For this review, take the finished solid that the model builds, in its own axes (mm). Face numbers are marked on the shaded views. A direction names the side the tool comes from. Round coordinates to 2 decimals unless told otherwise and drop trailing zeros. Loops run counter-clockwise (first coordinate to the right, second up) from the corner with the lowest first, then second, coordinate; pieces in that order, holes last.
1) Take a section at D-D (x = 24.5). State the section outline as (y, z) points, then the cut area to 3 significant figures.
2) Take a section at C-C (y = 42.5). State the section outline as (x, z) points.
3) Tool access review of the marked faces 1 and 2: name each direction out of +Z, -Z, +X, -X, +Y, -Y from which nothing blocks a thin tool from reaching the whole face with its end or side.
4) Take a section at A-A (z = 3). State the section outline as (x, y) points, then the cut area to 3 significant figures.
5) Insertion check: pin 1 (1.5 mm diameter, centred on x = 79, y = 78, fed in from +Z); pin 2 (12 mm diameter, centred on x = 22.5, y = 77.5, fed in from +Z). Each pin has a flat end and moves straight along its axis. Give the tip position at first contact, or say it passes through.
6) Take a section at B-B (x = 38). State the section outline as (y, z) points, then the cut area to 3 significant figures.
7) Mouldability with a two-part tool opening along X and no side actions: class the marked faces 3, 4 and 5 as pulls with the +X half, pulls with the -X half, needs draft (parallel to the pull), parting line crosses it, or undercut.
8) Wall thickness on L1, parallel to Y at x = 52, z = 10.25; L2, parallel to X at y = 70, z = 4; L3, parallel to Z at x = 44, y = 64.5: over which ranges is each line inside the solid? List them lowest first.
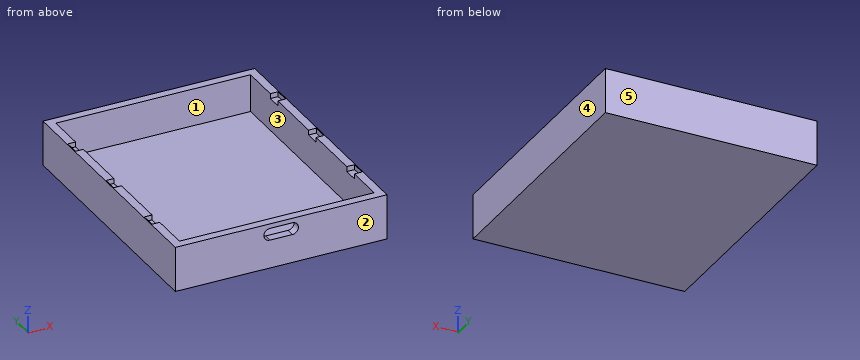
```python
from build123d import *

# Parameters (mm, degrees)
MODEL_W             = 84.74935
MODEL_H             = 103.79946
MODEL_W_2           = 77.94935
MODEL_H_2           = 96.99946
EXTRUDE_2_DEPTH     = 15
SKETCH_1_W          = 84.74935
SKETCH_1_H          = 103.79946
EXTRUDE_3_DEPTH     = 3
SKETCH_2_W          = 3.1
SKETCH_2_H          = 6
CUT_EXTRUDE_1_DEPTH = 2
CUT_EXTRUDE_3_DEPTH = 10


with BuildPart() as part:
    # Model → 凸台-拉伸2 (new body)
    with BuildSketch(Plane.XY):
        with Locations((38.194325, 47.88337)):
            Rectangle(MODEL_W, MODEL_H)
        with Locations((38.194325, 47.88337)):
            Rectangle(MODEL_W_2, MODEL_H_2, mode=Mode.SUBTRACT)
    extrude(amount=EXTRUDE_2_DEPTH)

    # 草图1 → 凸台-拉伸3 (add)
    with BuildSketch(Plane(origin=(0, 0, 0), x_dir=(-1, 0, 0), z_dir=(0, 0, -1))):
        with Locations((-38.194325, 47.88337)):
            Rectangle(SKETCH_1_W, SKETCH_1_H)
    extrude(amount=EXTRUDE_3_DEPTH)

    # 草图2 → 切除-拉伸1 (cut)
    with BuildSketch(Plane.XY.offset(15)):
        with Locations((-2.33035, 77.88337)):
            Rectangle(SKETCH_2_W, SKETCH_2_H)
        with Locations((-2.33035, 47.88337)):
            Rectangle(SKETCH_2_W, SKETCH_2_H)
        with Locations((-2.33035, 17.88337)):
            Rectangle(SKETCH_2_W, SKETCH_2_H)
        with Locations((78.719, 17.88337)):
            Rectangle(SKETCH_2_W, SKETCH_2_H)
        with Locations((78.719, 47.88337)):
            Rectangle(SKETCH_2_W, SKETCH_2_H)
        with Locations((78.719, 77.88337)):
            Rectangle(SKETCH_2_W, SKETCH_2_H)
    extrude(amount=-CUT_EXTRUDE_1_DEPTH, mode=Mode.SUBTRACT)

    # 草图4 → 切除-拉伸3 (cut)
    with BuildSketch(Plane.XZ.offset(7.21636)):
        with BuildLine():
            Line((33.694325, 13.169990539), (42.694325, 13.169990539))
            ThreePointArc((42.694325, 13.169990539), (45.094325, 10.769990539), (42.694325, 8.369990539))
            Line((42.694325, 8.369990539), (33.694325, 8.369990539))
            ThreePointArc((33.694325, 8.369990539), (31.294325, 10.769990539), (33.694325, 13.169990539))
        make_face()
    extrude(amount=-CUT_EXTRUDE_3_DEPTH, mode=Mode.SUBTRACT)


solid = part.part
```
Response:
1. outline: (-4.02, -3) - (99.78, -3) - (99.78, 15) - (96.38, 15) - (96.38, 0) - (-0.62, 0) - (-0.62, 15) - (-4.02, 15) - close
1. area: 413 mm2
2. outline: (-4.18, -3) - (80.57, -3) - (80.57, 15) - (77.17, 15) - (77.17, 0) - (-0.78, 0) - (-0.78, 15) - (-4.18, 15) - close
3. face 1: +Z
3. face 2: +Z, -Z, +X, -X, -Y
4. outline: (-4.18, -4.02) - (80.57, -4.02) - (80.57, 99.78) - (-4.18, 99.78) - close; hole (-0.78, -0.62) - (77.17, -0.62) - (77.17, 96.38) - (-0.78, 96.38) - close
4. area: 1,240 mm2
5. pin 1: stops at z = 13
5. pin 2: stops at z = 0
6. outline: (-4.02, -3) - (99.78, -3) - (99.78, 15) - (96.38, 15) - (96.38, 0) - (-0.62, 0) - (-0.62, 8.37) - (-4.02, 8.37) - close; (-4.02, 13.17) - (-0.62, 13.17) - (-0.62, 15) - (-4.02, 15) - close
6. area: 397 mm2
7. face 3: undercut
7. face 4: pulls with the +X half
7. face 5: needs draft
8. L1: y = -4.02 to -0.62, 96.38 to 99.78
8. L2: x = -4.18 to -0.78, 77.17 to 80.57
8. L3: z = -3 to 0
